Verification items for this drawing (mm, ordinates from the low corner). A direction names the side the tool comes from. Round coordinates to 2 decimals unless told otherwise and drop trailing zeros. Order: outer loops, then holes, each group sorted by start corner. A loop starts at its lowest first (then second) coordinate and runs counter-clockwise, first axis right, second up. Notation, with made-up numbers: (13.5, 37) - (49.5, 37) arc R25 ccw to (49.5, 76) - close; hole circle Ø5 at (-14, 85). An arc over 180 degrees is marked (long way). Use a Markdown table: item, result. Add a question column.
(1) Gauge pin test, flat ends, axial feed: P1, Ø3, axis at x = 99.5, y = 5, coming from the -Z side; P2, Ø7.5, axis at x = 63.5, z = 63.5, coming from the -Y side; P3, Ø5, axis at x = 68, y = 2.5, coming from the +Z side; P4, Ø1.5, axis at x = 95, y = 9.5, coming from the +Z side. Record the tip position at first contact, or that the pin passes through.
(2) Section check A-A on z = 63.5. Record the boundary of the cut face in (x, y).
(3) Section check B-B on x = 63.5. Record the boundary of the cut face in (y, z).
(4) Thickness scan on line 1 along X through (y, z) = (4.25, 47) (1 decimal); line 2 along Z through (x, y) = (53.5, 11.75) (1 decimal); line 3 along Z through (x, y) = (51, 9.5) (1 decimal). Record the ranges inside material, lowest first. Write a range as [from, to].
(5) Section check D-D on x = 16. Record the boundary of the cut face in (y, z), then the cut area to 3 significant figures.
(6) Section check C-C on y = 2.75. Record the boundary of the cut face in (x, z).
(7) Mould release check, pull along Z, two halves, no side actions. Record for the marked faces 1, 2 and 3: released by +Z, released by -Z, zero draft, split by the parting line, or undercut.
(8) Access from +Z, -Z, +X, -X, +Y, -Y to the whole of each face (thin tool, end or side, straight path). Record for the marked faces 4 and 5.
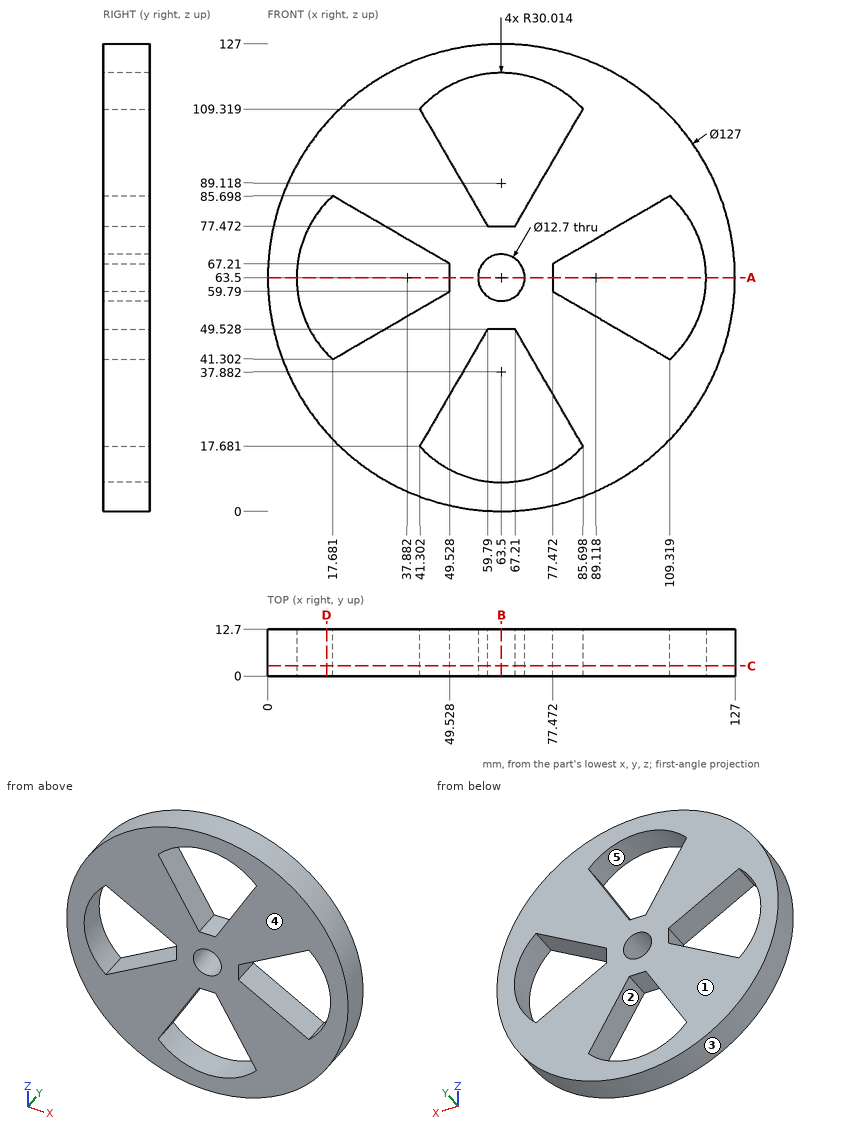
Check sheet entries:
| question | item | result |
|---|---|---|
| 1 | P1 | stops at z = 10.19 |
| 1 | P2 | passes through |
| 1 | P3 | stops at z = 126.97 |
| 1 | P4 | stops at z = 119.06 |
| 2 | outline | (0, 0) - (7.87, 0) - (7.87, 12.7) - (0, 12.7) - close; (49.53, 0) - (57.15, 0) - (57.15, 12.7) - (49.53, 12.7) - close; (69.85, 0) - (77.47, 0) - (77.47, 12.7) - (69.85, 12.7) - close; (119.13, 0) - (127, 0) - (127, 12.7) - (119.13, 12.7) - close |
| 3 | outline | (0, 0) - (12.7, 0) - (12.7, 7.87) - (0, 7.87) - close; (0, 49.53) - (12.7, 49.53) - (12.7, 57.15) - (0, 57.15) - close; (0, 69.85) - (12.7, 69.85) - (12.7, 77.47) - (0, 77.47) - close; (0, 119.13) - (12.7, 119.13) - (12.7, 127) - (0, 127) - close |
| 4 | line 1 | x = [2.2, 12.8], [27.5, 58.3], [68.7, 99.5], [114.2, 124.8] |
| 4 | line 2 | z = [0.8, 9.6], [38.7, 88.3], [117.4, 126.2] |
| 4 | line 3 | z = [1.2, 10.6], [34.4, 92.6], [116.4, 125.8] |
| 5 | outline | (0, 21.36) - (12.7, 21.36) - (12.7, 42.96) - (0, 42.96) - close; (0, 84.04) - (12.7, 84.04) - (12.7, 105.64) - (0, 105.64) - close |
| 5 | area | 549 mm2 |
| 6 | outline | circle Ø127 at (63.5, 63.5); hole (17.68, 41.3) - (49.53, 59.79) - (49.53, 67.21) - (17.68, 85.7) arc R30.01 ccw to start; hole (41.3, 17.68) arc R30.01 ccw to (85.7, 17.68) - (67.21, 49.53) - (59.79, 49.53) - close; hole (41.3, 109.32) - (59.79, 77.47) - (67.21, 77.47) - (85.7, 109.32) arc R30.01 ccw to start; hole circle Ø12.7 at (63.5, 63.5); hole (77.47, 59.79) - (109.32, 41.3) arc R30.01 ccw to (109.32, 85.7) - (77.47, 67.21) - close |
| 7 | face 1 | zero draft |
| 7 | face 2 | undercut |
| 7 | face 3 | split by the parting line |
| 8 | face 4 | +Z, -Z, +X, -X, -Y |
| 8 | face 5 | +Y, -Y |
